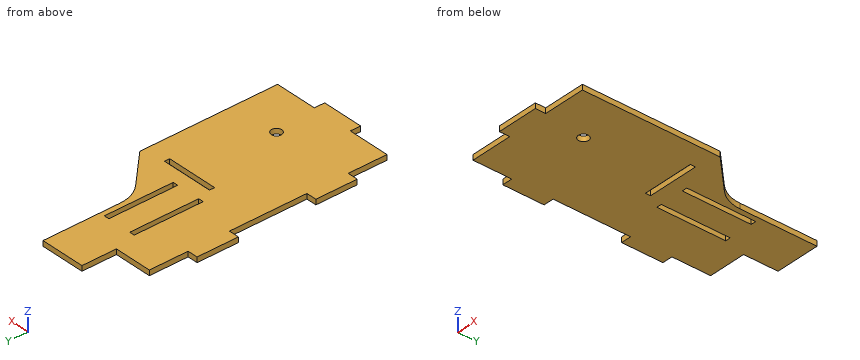
from build123d import *

# Parameters (mm, degrees)
BASESHAPE_DEPTH   = 3
SKETCH2_R         = 3
SHAFTHOLES_DEPTH  = 157.147366292
SKETCH4_W         = 6
SKETCH4_H         = 24
SKETCH4_W_2       = 24
SKETCH4_H_2       = 6
FINGERS_DEPTH     = 3
SKETCH5_W         = 30
SKETCH5_H         = 3
SKETCH5_W_2       = 3
SKETCH5_H_2       = 40
GROOVES_DEPTH     = 160.040875249
CHAMFER1_SIZE     = 25
FILLET2_R         = 20
SKETCH6_W         = 26
SKETCH6_H         = 3
MARBLECHUTE_DEPTH = 20


with BuildPart() as part:
    # Sketch1 → BaseShape (new body)
    with BuildSketch(Plane.XY):
        Polygon((-73, 138), (-73, 0), (0, 0), (0, 77), (-31, 77), (-31, 138), align=None)
    extrude(amount=BASESHAPE_DEPTH)

    # Sketch2 → ShaftHoles (cut, through all)
    with BuildSketch(Plane.XY.offset(3)):
        with Locations((-28, 25)):
            Circle(SKETCH2_R)
    extrude(amount=-SHAFTHOLES_DEPTH, mode=Mode.SUBTRACT)

    # Sketch4 → Fingers (add)
    with BuildSketch(Plane.XY.offset(3)):
        Polygon((0, 77), (-31, 77), (-31, 80), (-31, 138), (-25, 138), (-25, 80), (0, 80), align=None)
        with Locations((-76, 103.5)):
            Rectangle(SKETCH4_W, SKETCH4_H)
        with Locations((-76, 34.5)):
            Rectangle(SKETCH4_W, SKETCH4_H)
        with Locations((-36.5, -3)):
            Rectangle(SKETCH4_W_2, SKETCH4_H_2)
    extrude(amount=-FINGERS_DEPTH)

    # Sketch5 → Grooves (cut, through all)
    with BuildSketch(Plane.XY.offset(3)):
        with Locations((-28, 75.5)):
            Rectangle(SKETCH5_W, SKETCH5_H)
        with Locations((-46.5, 105)):
            Rectangle(SKETCH5_W_2, SKETCH5_H_2)
        with Locations((-29.5, 105)):
            Rectangle(SKETCH5_W_2, SKETCH5_H_2)
    extrude(amount=-GROOVES_DEPTH, mode=Mode.SUBTRACT)

    # Chamfer1
    chamfer1_edges = [part.edges().sort_by_distance(p)[0] for p in [
        (-25, 80, 1.5),
    ]]
    chamfer(chamfer1_edges, length=CHAMFER1_SIZE - 0.0001)  # a hair under: the kernel refuses the full size

    # Fillet2
    fillet2_edges = [part.edges().sort_by_distance(p)[0] for p in [
        (-25, 104.9999, 1.5),
    ]]
    fillet(fillet2_edges, radius=FILLET2_R)

    # Sketch6 → MarbleChute (add)
    with BuildSketch(Plane(origin=(0, 138, 0), x_dir=(1, 0, 0), z_dir=(0, 1, 0))):
        with Locations((-38, -1.5)):
            Rectangle(SKETCH6_W, SKETCH6_H)
    extrude(amount=MARBLECHUTE_DEPTH)


solid = part.part
Can you work these out from the model? Positions are in its coordinate system, mm. Round coordinates to 2 decimals unless told otherwise and drop trailing zeros. Loops run counter-clockwise (first coordinate to the right, second up) from the corner with the lowest first, then second, coordinate; pieces in that order, holes last. Notation, with made-up numbers: (-22, 53) - (27, 53) arc R20 cw to (27, 82) - close; hole circle Ø3 at (64.25, -30.75). An arc over 180 degrees is marked (long way). Use CSV: the item, a comma, the result in double quotes. Start each with the question number.
1) If we section it at A-A on x = -34.5: Write out the boundary of the cut face in (y, z), plus the area to 3 significant figures.
2) For pin 1 Ø1.5 at (y, z) = (-2.5, 1) entering from +X; pin 2 Ø1.5 at (y, z) = (114, 2) entering from +X; pin 3 Ø1.5 at (y, z) = (6.5, 2) entering from -X; pin 4 Ø3.5 at (x, y) = (-28, 25) entering from +Z, each with a flat end and sliding along its axis, tell me the tip position at first contact or that it passes through.
3) Please list where these lines run through material, in increasing order: probe 1 along X at (y, z) = (112, 2); probe 2 along Y at (x, z) = (-30.5, 1.7); probe 3 along X at (y, z) = (109.5, 2.05). Write a range as [from, to].
4) If we section it at B-B on y = 25: Write out the boundary of the cut face in (x, z).
5) If we section it at C-C on y = 119: Write out the boundary of the cut face in (x, z).
6) If we section it at D-D on z = 1.8: Count the separate pieces of the cut face and the enclosed holes in it, plus the area to 3 significant figures.
Geometry results:
1,outline,"(-6, 0) - (74, 0) - (74, 3) - (-6, 3) - close; (77, 0) - (158, 0) - (158, 3) - (77, 3) - close"
1,area,"483 mm2"
2,pin 1,"stops at x = -24.5"
2,pin 2,"stops at x = -25"
2,pin 3,"stops at x = -73"
2,pin 4,"passes through"
3,probe 1,"x = [-79, -48], [-45, -31], [-28, -24.96]"
3,probe 2,"y = [-6, 23.34], [26.66, 74], [77, 85], [125, 158]"
3,probe 3,"x = [-79, -48], [-45, -31], [-28, -24.64]"
4,outline,"(-79, 0) - (-31, 0) - (-31, 3) - (-79, 3) - close; (-25, 0) - (0, 0) - (0, 3) - (-25, 3) - close"
5,outline,"(-73, 0) - (-48, 0) - (-48, 3) - (-73, 3) - close; (-45, 0) - (-31, 0) - (-31, 3) - (-45, 3) - close; (-28, 0) - (-25, 0) - (-25, 3) - (-28, 3) - close"
6,separate pieces,"1"
6,enclosed holes,"4"
6,area,"9,540 mm2"
